Work out the finished part from the listing and answer in its coordinate system (mm). Face numbers are marked on the shaded views. A direction names the side the tool comes from. Give positions to 0.01 mm unless a question says otherwise; leave off trailing zeros. Order: outer loops, then holes, each group sorted by start corner. A loop starts at its lowest first (then second) coordinate and runs counter-clockwise, first axis right, second up. Notation, with made-up numbers: (-38.5, 42.25) -> (16.5, 42.25) arc R16 ccw to (16.5, 70.25) -> close; hole circle Ø1 at (13.5, 86). An arc over 180 degrees is marked (long way). Answer as CSV lines item,"result". Start each with the question number.
1. A cutting plane is placed at C-C (x = 28). Give the vertices of the cut face in (y, z), then the cut area to 3 significant figures.
2. For the marked faces 5 and 6, determine the directions among +Z, -Z, +X, -X, +Y, -Y from which every point of the face is accessible in a straight line to the end or side of a thin tool.
3. Find the intervals of material crossed by L1, parallel to X at y = -3, z = 5; L2, parallel to Y at x = 0, z = 2; L3, parallel to Z at x = -5, y = -19.5, in increasing order.
4. A cutting plane is placed at B-B (x = 0). Give the vertices of the cut face in (y, z), then the cut area to 3 significant figures.
5. A cutting plane is placed at A-A (y = 0). Give the vertices of the cut face in (x, z), then the cut area to 3 significant figures.
6. Flat-ended cylindrical pins translate along their axes: pin 1 (5 mm diameter, centred on x = 14.5, y = 23.5, fed in from +Z); pin 2 (2 mm diameter, centred on y = -10.5, z = 5, fed in from -X); pin 3 (1.3 mm diameter, centred on y = 1, z = 6, fed in from +X). Find the tip coordinate at first contact, or state that the pin passes through.
7. For a pull along X with two mould halves and no side action, classify the marked faces 1, 2, 3 and 4 as released by +X, released by -X, zero draft, split by the parting line, or undercut.
from build123d import *

# Parameters (mm, degrees)
F2_R     = 7.9375
F2_R_2   = 2.778125
F3_DEPTH = 25.4
F4_DEPTH = 10.16


with BuildPart() as f1:
    # F0 (on Front) → F1 (revolve)
    with BuildSketch(Plane.XZ):
        Polygon((-31.75, 0), (0, 0), (0, 13.890625), (-11.90625, 13.890625), (-19.05, 7.9375), (-31.75, 7.9375), align=None)
    revolve(axis=Axis((0, 0, 6.945312), (0, 0, 1)))

    # F2 (on face) → F3 (cut)
    with BuildSketch(Plane.XY.offset(13.890625)):
        Circle(F2_R)
        with Locations((-11.90625, 20.62223)):
            Circle(F2_R_2)
        with Locations((11.90625, 20.62223)):
            Circle(F2_R_2)
        with BuildLine():
            ThreePointArc((26.590625, 0), (23.8125, 2.778125), (21.034375, 0))
            ThreePointArc((21.034375, 0), (23.8125, -2.778125), (26.590625, 0))
        make_face()
        with Locations((11.90625, -20.62223)):
            Circle(F2_R_2)
        with Locations((-11.90625, -20.62223)):
            Circle(F2_R_2)
        with Locations((-23.8125, 0)):
            Circle(F2_R_2)
    extrude(amount=-F3_DEPTH, mode=Mode.SUBTRACT)

    # F2 (on face) → F4 (cut)
    with BuildSketch(Plane.XY.offset(13.890625)):
        Polygon((-16.98625, 23.555169), (-16.98625, 17.689291), (-11.90625, 14.756351), (-6.82625, 17.689291), (-6.82625, 23.555169), (-11.90625, 26.488109), align=None)
        with Locations((-11.90625, 20.62223)):
            Circle(F2_R_2, mode=Mode.SUBTRACT)
        Polygon((11.90625, 26.488109), (6.82625, 23.555169), (6.82625, 17.689291), (11.90625, 14.756351), (16.98625, 17.689291), (16.98625, 23.555169), align=None)
        with Locations((11.90625, 20.62223)):
            Circle(F2_R_2, mode=Mode.SUBTRACT)
        Polygon((18.7325, 2.932939), (18.7325, 0), (18.7325, -2.932939), (23.8125, -5.865879), (28.8925, -2.932939), (28.8925, 2.932939), (23.8125, 5.865879), align=None)
        with BuildLine():
            ThreePointArc((26.590625, 0), (23.8125, -2.778125), (21.034375, 0))
            ThreePointArc((21.034375, 0), (23.8125, 2.778125), (26.590625, 0))
        make_face(mode=Mode.SUBTRACT)
        Polygon((16.98625, -23.555169), (16.98625, -17.689291), (11.90625, -14.756351), (6.82625, -17.689291), (6.82625, -23.555169), (11.90625, -26.488109), align=None)
        with Locations((11.90625, -20.62223)):
            Circle(F2_R_2, mode=Mode.SUBTRACT)
        Polygon((-11.90625, -26.488109), (-6.82625, -23.555169), (-6.82625, -17.689291), (-11.90625, -14.756351), (-16.98625, -17.689291), (-16.98625, -23.555169), align=None)
        with Locations((-11.90625, -20.62223)):
            Circle(F2_R_2, mode=Mode.SUBTRACT)
        Polygon((-28.8925, -2.932939), (-23.8125, -5.865879), (-18.7325, -2.932939), (-18.7325, 2.932939), (-23.8125, 5.865879), (-28.8925, 2.932939), align=None)
        with Locations((-23.8125, 0)):
            Circle(F2_R_2, mode=Mode.SUBTRACT)
    extrude(amount=-F4_DEPTH, mode=Mode.SUBTRACT)


solid = f1.part
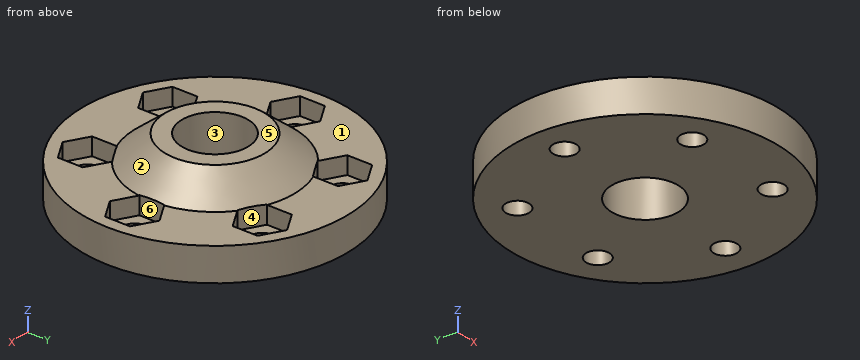
Answer sheet:
1,outline,"(-14.97, 0) -> (14.97, 0) -> (14.97, 7.94) -> (3.45, 7.94) -> (3.45, 3.73) -> (-3.45, 3.73) -> (-3.45, 7.94) -> (-14.97, 7.94) -> close"
1,area,"209 mm^2"
2,face 5,"+Z, +X, -X, +Y, -Y"
2,face 6,"+Z"
3,L1,"x = -31.61 to -28.78, -18.85 to -7.35, 7.35 to 18.85, 28.78 to 31.61"
3,L2,"y = -31.75 to -7.94, 7.94 to 31.75"
3,L3,"z = 0 to 7.94"
4,outline,"(-31.75, 0) -> (-7.94, 0) -> (-7.94, 13.89) -> (-11.91, 13.89) -> (-19.05, 7.94) -> (-31.75, 7.94) -> close; (7.94, 0) -> (31.75, 0) -> (31.75, 7.94) -> (19.05, 7.94) -> (11.91, 13.89) -> (7.94, 13.89) -> close"
4,area,"468 mm^2"
5,outline,"(-31.75, 0) -> (-26.59, 0) -> (-26.59, 3.73) -> (-28.89, 3.73) -> (-28.89, 7.94) -> (-31.75, 7.94) -> close; (-21.03, 0) -> (-7.94, 0) -> (-7.94, 13.89) -> (-11.91, 13.89) -> (-18.73, 8.2) -> (-18.73, 3.73) -> (-21.03, 3.73) -> close; (7.94, 0) -> (21.03, 0) -> (21.03, 3.73) -> (18.73, 3.73) -> (18.73, 8.2) -> (11.91, 13.89) -> (7.94, 13.89) -> close; (26.59, 0) -> (31.75, 0) -> (31.75, 7.94) -> (28.89, 7.94) -> (28.89, 3.73) -> (26.59, 3.73) -> close"
5,area,"341 mm^2"
6,pin 1,"stops at z = 7.94"
6,pin 2,"stops at x = -30.3"
6,pin 3,"stops at x = 31.75"
7,face 1,"zero draft"
7,face 2,"split by the parting line"
7,face 3,"undercut"
7,face 4,"undercut"
